Source: CAD feature listing. Evaluate the final solid. Frame: model axes, mm. A direction names the side the tool comes from. Coordinates: 2 decimals unless noted, no trailing zeros. Loops run counter-clockwise (first coordinate to the right, second up) from the corner with the lowest first, then second, coordinate; pieces in that order, holes last. Notation, with made-up numbers: M -37,68 L -24,68 A7 cw -24,79 Z; hole C 66,25.25 d9. An arc over 180 degrees is marked long. One line per question, with ' | ' between items. Start each with the question number.
1. Pin query (flat end, axial travel): P1, Ø3, axis at x = -8.5, z = -9, coming from the -Y side. Return the tip coordinate at first contact, or that it passes through.
2. Mould query, pull axis Z, two halves, no side actions, for faces 3 (the cylindrical face through (-15.023, -1.183, 16.152)), 4 (the cylindrical face through (-18.797, 0.296, 21.959)), 5 (the cylindrical face through (11.4, 0.3, -10.8)), 6 (the flat face through (-16, -2.4, 0)). Classes: pulls with the +Z half, pulls with the -Z half, needs draft (parallel to the pull), parting line crosses it, or undercut.
3. Section query C-C, the plane x = 0. Output: boundary loops of the cut face in (y, z).
4. Section query A-A, the plane y = -1.4. State how many separate pieces and enclosed holes the cut face has, and give its area (3 significant figures).
5. Ray query, probe 1 along Z at (x, y) = (1, -0.35); probe 2 along Y at (x, z) = (12, 1); probe 3 along X at (y, z) = (-1.35, -17.5). Return the intervals inside material, ascending.
6. Section query B-B, the plane z = 0. Output: boundary loops of the cut face in (x, y), and give its area (3 significant figures).
7. Access query for faces 1 (the cylindrical face through (15.1, -1.18, 16.09)), 2 (the cylindrical face through (-18.859, 0.296, -21.897)). Directions: +Z, -Z, +X, -X, +Y, -Y. A direction counts if a zero-diameter tool reaches every point of the face in a straight line with its end or side. Return the directions, or none.
8. Section query D-D, the plane z = 17. Output: boundary loops of the cut face in (x, y), and give its area (3 significant figures).
```python
from build123d import *

# Parameters (mm, degrees)
BOSS_EXTRUDE1_DEPTH = 0.6
SKETCH3_R           = 2
CUT_EXTRUDE1_DEPTH  = 10
SKETCH4_R           = 1.15
BOSS_EXTRUDE3_DEPTH = 3


with BuildPart() as part:
    # Sketch2 → Boss-Extrude1 (new body)
    with BuildSketch(Plane(origin=(0, 0, 0), x_dir=(1, 0, 0), z_dir=(0, 1, 0))):
        with BuildLine():
            Line((-16, 23.1), (16, 23.1))
            ThreePointArc((16, 23.1), (18.828427125, 21.928427125), (20, 19.1))
            Line((20, 19.1), (20, -19.1))
            ThreePointArc((20, -19.1), (18.828427125, -21.928427125), (16, -23.1))
            Line((16, -23.1), (-16, -23.1))
            ThreePointArc((-16, -23.1), (-18.828427125, -21.928427125), (-20, -19.1))
            Line((-20, -19.1), (-20, 19.1))
            ThreePointArc((-20, 19.1), (-18.828427125, 21.928427125), (-16, 23.1))
        make_face()
    extrude(amount=BOSS_EXTRUDE1_DEPTH)

    # Sketch3 → Cut-Extrude1 (cut)
    with BuildSketch(Plane(origin=(0, 0.6, 0), x_dir=(1, 0, 0), z_dir=(0, 1, 0))):
        with Locations(Location((10.84244602, -11.278395934, 0), (0, 0, 270))):
            Circle(SKETCH3_R)
        with Locations(Location((10.84244602, 0.721604066, 0), (0, 0, 270))):
            Circle(SKETCH3_R)
        with Locations(Location((10.84244602, 12.721604066, 0), (0, 0, 270))):
            Circle(SKETCH3_R)
    extrude(amount=-CUT_EXTRUDE1_DEPTH, mode=Mode.SUBTRACT)

    # Sketch4 → Boss-Extrude3 (add)
    with BuildSketch(Plane(origin=(0, 0.6, 0), x_dir=(1, 0, 0), z_dir=(0, 1, 0))):
        with Locations(Location((15.8, 17, 0), (0, 0, 270))):
            Circle(SKETCH4_R)
        with Locations(Location((0, 17, 0), (0, 0, 270))):
            Circle(SKETCH4_R)
        with Locations(Location((-15.8, 17, 0), (0, 0, 270))):
            Circle(SKETCH4_R)
        with Locations(Location((0, 0, 0), (0, 0, 270))):
            Circle(SKETCH4_R)
        with Locations(Location((-15.8, 0, 0), (0, 0, 270))):
            Circle(SKETCH4_R)
        with Locations(Location((0, -17, 0), (0, 0, 270))):
            Circle(SKETCH4_R)
        with Locations(Location((-15.8, -17, 0), (0, 0, 270))):
            Circle(SKETCH4_R)
        with Locations(Location((15.8, 0, 0), (0, 0, 270))):
            Circle(SKETCH4_R)
        with Locations(Location((15.8, -17, 0), (0, 0, 270))):
            Circle(SKETCH4_R)
    extrude(amount=-BOSS_EXTRUDE3_DEPTH)


solid = part.part
```
Taken from the geometry:
1) P1: y = 0
2) face 3: undercut | face 4: pulls with the +Z half | face 5: undercut | face 6: needs draft
3) outline: M -2.4,-18.15 L 0,-18.15 L 0,-23.1 L 0.6,-23.1 L 0.6,23.1 L 0,23.1 L 0,18.15 L -2.4,18.15 L -2.4,15.85 L 0,15.85 L 0,1.15 L -2.4,1.15 L -2.4,-1.15 L 0,-1.15 L 0,-15.85 L -2.4,-15.85 Z
4) separate pieces: 9 | enclosed holes: 0 | area: 37.4 mm^2
5) probe 1: -17.57 to -16.43, -0.57 to 0.57, 16.43 to 17.57 | probe 2: 0 to 0.6 | probe 3: -16.84 to -14.76, -1.04 to 1.04, 14.76 to 16.84
6) outline: M -20,0 L -16.95,0 L -16.95,-2.4 L -14.65,-2.4 L -14.65,0 L -1.15,0 L -1.15,-2.4 L 1.15,-2.4 L 1.15,0 L 8.98,0 L 8.98,0.6 L -20,0.6 Z; M 12.71,0 L 14.65,0 L 14.65,-2.4 L 16.95,-2.4 L 16.95,0 L 20,0 L 20,0.6 L 12.71,0.6 Z | area: 38.3 mm^2
7) face 1: -Y | face 2: -Z, -X, +Y, -Y
8) outline: M -20,0 L -16.95,0 L -16.95,-2.4 L -14.65,-2.4 L -14.65,0 L -1.15,0 L -1.15,-2.4 L 1.15,-2.4 L 1.15,0 L 14.65,0 L 14.65,-2.4 L 16.95,-2.4 L 16.95,0 L 20,0 L 20,0.6 L -20,0.6 Z | area: 40.6 mm^2
